```python
from build123d import *

# Parameters (mm, degrees)
SKETCH1_W           = 33
SKETCH1_H           = 7.5
BOSS_EXTRUDE1_DEPTH = 0.1
SKETCH2_W           = 5.2
SKETCH2_H           = 6.9
BOSS_EXTRUDE2_DEPTH = 2.6
CHAMFER1_SIZE       = 0.5
SKETCH3_R           = 1.05
CUT_EXTRUDE1_DEPTH  = 2.6


with BuildPart() as part:
    # Sketch1 → Boss-Extrude1 (new body)
    with BuildSketch(Plane(origin=(0, 0, 0), x_dir=(1, 0, 0), z_dir=(0, 1, 0))):
        with Locations((16.5, 3.75)):
            Rectangle(SKETCH1_W, SKETCH1_H)
    extrude(amount=BOSS_EXTRUDE1_DEPTH)

    # Sketch2 → Boss-Extrude2 (add)
    with BuildSketch(Plane(origin=(0, 0.1, 0), x_dir=(1, 0, 0), z_dir=(0, 1, 0))):
        with Locations((0.2, 3.75)):
            Rectangle(SKETCH2_W, SKETCH2_H)
    extrude(amount=BOSS_EXTRUDE2_DEPTH)

    # Chamfer1
    chamfer1_edges = [part.edges().sort_by_distance(p)[0] for p in [
        (-1.2, 0.1, -0.3),
        (-1.2, 0.1, -7.2),
    ]]
    chamfer(chamfer1_edges, length=CHAMFER1_SIZE)

    # Sketch3 → Cut-Extrude1 (cut)
    with BuildSketch(Plane.XZ):
        with Locations(Location((5.5, -3.75, 0), (0, 0, 270))):
            Circle(SKETCH3_R)
        with Locations(Location((16, -3.75, 0), (0, 0, 270))):
            Circle(SKETCH3_R)
    extrude(amount=-CUT_EXTRUDE1_DEPTH, mode=Mode.SUBTRACT)


solid = part.part
```
Build history of the part. All positions in model axes, mm. A direction names the side the tool comes from. Coordinates: 2 decimals unless noted, no trailing zeros. Write each loop counter-clockwise with the first axis right and the second up, starting at its lowest first coordinate (ties: lowest second). Pieces come first, ordered by that corner, then holes.
1. 3-axis set-ups, long thin cutter, end or side, ignore diameter. For faces 1 (the flat face through (0, 1, -0.3)), 2 (the flat face through (2.8, 1, -4)), 3 (the flat face through (-2.4, 1, -4)), 4 (the flat face through (0, 1, -7.2)), 5 (the flat face through (-1, 0.1, -4)): which of +Z, -Z, +X, -X, +Y, -Y reach the whole face in a straight line?
Answer block:
face 1: +Z, +X, -X, +Y
face 2: +Z, -Z, +X, +Y
face 3: +Z, -Z, -X, +Y, -Y
face 4: -Z, +X, -X, +Y
face 5: +Z, -Z, -X, -Y
2. Drop flat-ended pins along their axis: pin 1 (1.3 mm diameter, centred on x = -0.5, y = 2, fed in from -Z); pin 2 (2.5 mm diameter, centred on x = 16, z = -3.75, fed in from +Y); pin 3 (1.3 mm diameter, centred on y = 2, z = -3.5, fed in from +X). Give the stop position or say it passes through.
Answer block:
pin 1: stops at z = -7.2
pin 2: stops at y = 0.1
pin 3: stops at x = 2.8
3. Band-saw the part on C-C, the plane z = -6. Give the cut face in (x, y), and give its area (3 significant figures).
Answer block:
outline: (-2.4, 0.1) - (0, 0.1) - (0, 0) - (33, 0) - (33, 0.1) - (2.8, 0.1) - (2.8, 2.7) - (-2.4, 2.7) - close
area: 16.8 mm2
4. Band-saw the part on D-D, the plane y = 1.25. Give the cut face in (x, z).
Answer block:
outline: (-2.4, -7.2) - (2.8, -7.2) - (2.8, -0.3) - (-2.4, -0.3) - close
5. Band-saw the part on A-A, the plane z = -3.75. Give the cut face in (x, y), and give its area (3 significant figures).
Answer block:
outline: (-2.4, 0.1) - (0, 0.1) - (0, 0) - (4.45, 0) - (4.45, 0.1) - (2.8, 0.1) - (2.8, 2.7) - (-2.4, 2.7) - close; (6.55, 0) - (14.95, 0) - (14.95, 0.1) - (6.55, 0.1) - close; (17.05, 0) - (33, 0) - (33, 0.1) - (17.05, 0.1) - close
area: 16.4 mm2
6. Drill centre lines: probe 1 along X at (y, z) = (0.05, -3.75); probe 2 along X at (y, z) = (0.7, -2.5); probe 3 along Z at (x, y) = (2, 1.75). Where is each one in solid material? Low to high.
Answer block:
probe 1: x = 0 to 4.45, 6.55 to 14.95, 17.05 to 33
probe 2: x = -2.4 to 2.8
probe 3: z = -7.2 to -0.3
7. Band-saw the part on B-B, the plane x = 5.5. Give the cut face in (y, z), and give its area (3 significant figures).
Answer block:
outline: (0, -7.5) - (0.1, -7.5) - (0.1, -4.8) - (0, -4.8) - close; (0, -2.7) - (0.1, -2.7) - (0.1, 0) - (0, 0) - close
area: 0.540 mm2
